For this review, take the finished solid that the model builds, in its own axes (mm). A direction names the side the tool comes from. Give positions to 0.01 mm unless a question says otherwise; leave off trailing zeros. Order: outer loops, then holes, each group sorted by start corner. A loop starts at its lowest first (then second) coordinate and runs counter-clockwise, first axis right, second up.
from build123d import *

# Parameters (mm, degrees)
CYLINDER003_R          = 1.7
CYLINDER003_DEPTH      = 18
CYLINDER003_ROLL_ANGLE = 90.0000000001
CYLINDER002_R          = 3.5
CYLINDER002_DEPTH      = 35
CYLINDER004_R          = 1.5
CYLINDER004_DEPTH      = 40
SKETCH_R               = 4
PAD_DEPTH              = 20
CYLINDER001_R          = 19
CYLINDER001_DEPTH      = 30
CYLINDER001_ROLL_ANGLE = 90.0000000001
CYLINDER_R             = 26.62
CYLINDER_DEPTH         = 40
CYLINDER_ROLL_ANGLE    = 90.0000000001
CUT002_ROLL_ANGLE      = -20


with BuildPart() as cilindro003:
    # Cylinder003 → Cylinder003 (new body)
    with BuildSketch(Plane.XY):
        Circle(CYLINDER003_R)
    extrude(amount=CYLINDER003_DEPTH)


with BuildPart() as cilindro003_1:
    # Cylinder003 roll: moved
    add(cilindro003.part.rotate(Axis((0, 0, 0), (1, 0, 0)), CYLINDER003_ROLL_ANGLE))


with BuildPart() as cilindro003_2:
    # Cylinder003 placement: moved
    add(cilindro003_1.part)


with BuildPart() as cilindro002:
    # Cylinder002 → Cylinder002 (new body)
    with BuildSketch(Plane(origin=(0, -13, 5), x_dir=(1, 0, 0), z_dir=(0, 0, 1))):
        Circle(CYLINDER002_R)
    extrude(amount=CYLINDER002_DEPTH)


with BuildPart() as fusion001:
    # Cylinder004 → Cylinder004 (new body)
    with BuildSketch(Plane(origin=(0, -13, 0), x_dir=(1, 0, 0), z_dir=(0, 0, 1))):
        Circle(CYLINDER004_R)
    extrude(amount=CYLINDER004_DEPTH)

    # Fusion001: union Cilindro003, Cilindro002
    add(cilindro003_2.part)
    add(cilindro002.part)


with BuildPart() as pad:
    # Sketch → Pad (new body, symmetric)
    with BuildSketch(Plane.XZ):
        with Locations((0, 26.6209914966)):
            Circle(SKETCH_R)
        with Locations((14.3923946042, 22.395003144)):
            Circle(SKETCH_R)
        with Locations((24.2153056134, 11.0587595287)):
            Circle(SKETCH_R)
        with Locations((26.3500281875, -3.7885620995)):
            Circle(SKETCH_R)
        with Locations((20.1188029925, -17.4330420298)):
            Circle(SKETCH_R)
        with Locations((7.5, -25.5426542917)):
            Circle(SKETCH_R)
        with Locations((-7.5, -25.5426542917)):
            Circle(SKETCH_R)
        with Locations((-26.3500281875, -3.7885620995)):
            Circle(SKETCH_R)
        with Locations((-24.2153056134, 11.0587595287)):
            Circle(SKETCH_R)
        with Locations((-14.3923946042, 22.395003144)):
            Circle(SKETCH_R)
        with Locations((-20.1188029925, -17.4330420298)):
            Circle(SKETCH_R)
    extrude(amount=PAD_DEPTH, both=True)


with BuildPart() as cilindro001:
    # Cylinder001 → Cylinder001 (new body)
    with BuildSketch(Plane.XY):
        Circle(CYLINDER001_R)
    extrude(amount=CYLINDER001_DEPTH)


with BuildPart() as cilindro001_1:
    # Cylinder001 roll: moved
    add(cilindro001.part.rotate(Axis((0, 0, 0), (1, 0, 0)), CYLINDER001_ROLL_ANGLE))


with BuildPart() as cilindro001_2:
    # Cylinder001 placement: moved
    add(cilindro001_1.part.moved(Location((0, 20, 0))))


with BuildPart() as cut002:
    # Cylinder → Cylinder (new body)
    with BuildSketch(Plane.XY):
        Circle(CYLINDER_R)
    extrude(amount=CYLINDER_DEPTH)


with BuildPart() as cut002_1:
    # Cylinder roll: moved
    add(cut002.part.rotate(Axis((0, 0, 0), (1, 0, 0)), CYLINDER_ROLL_ANGLE))


with BuildPart() as cut002_2:
    # Cylinder placement: moved
    add(cut002_1.part.moved(Location((0, 20, 0))))

    # Cut: cut Cilindro001
    add(cilindro001_2.part, mode=Mode.SUBTRACT)

    # Cut001: cut Pad
    add(pad.part, mode=Mode.SUBTRACT)

    # Cut002: cut Fusion001
    add(fusion001.part, mode=Mode.SUBTRACT)


with BuildPart() as cut002_3:
    # Cut002 roll: moved
    add(cut002_2.part.rotate(Axis((0, 0, 0), (1, 0, 0)), CUT002_ROLL_ANGLE))


with BuildPart() as cut002_4:
    # Cut002 placement: moved
    add(cut002_3.part)


with BuildPart() as part_mirroring008:
    # Part__Mirroring008: instance of Cut002
    add(cut002_4.part.mirror(Plane(origin=(0, 45, 0), x_dir=(1, 0, 0), z_dir=(0, 1, 0))))


solid = part_mirroring008.part
1) Tool access review of faces 1 (the face through (-14.434, 97.387, -21.114)), 2 (the face through (-0.27, 100.76, -0.33)): name each direction out of +Z, -Z, +X, -X, +Y, -Y from which nothing blocks a thin tool from reaching the whole face with its end or side.
Answer sheet:
face 1: -Z, -X, +Y
face 2: none
2) Draft analysis for pull direction Y (two halves, no side actions). For faces 3 (the face through (-7.45, 81, 23.92)), 4 (the face through (-0.373, 108.718, 7.047)), 5 (the face through (10.214, 79.625, 13.273)), state which applies: +Y half, -Y half, draft (parallel to the pull), parting line (faces both ways), or undercut.
Answer sheet:
face 3: -Y half
face 4: +Y half
face 5: undercut
3) We need section A-A on x = 8.5. Give the boundary of the cut face in (y, z), then the cut area to 3 significant figures.
Answer sheet:
outline: (62.58, 16.86) - (65.39, 9.13) - (93.59, 19.39) - (105.21, -12.55) - (77.02, -22.81) - (78.62, -27.2) - (116.21, -13.52) - (100.17, 30.55) - close
area: 856 mm2
4) To check wall thickness, follow line 1 (X direction, y = 85, z = -8.5); line 2 (X direction, y = 101, z = -2); line 3 (Z direction, x = 1, y = 88.5). State the ranges of each line that lie inside material, in increasing order.
Answer sheet:
line 1: x = -23.22 to -17.93, 17.93 to 23.22
line 2: x = -22.81 to -18.14, 18.14 to 22.81
line 3: z = -28.85 to -20.74, 19.65 to 23.66
5) Clearance check with flat-ended pins moving along their axes: pin 1 (3 mm diameter, centred on y = 86, z = -25.5, fed in from -X); pin 2 (3 mm diameter, centred on x = 20, z = -6, fed in from +Y); pin 3 (3 mm diameter, centred on x = 0, z = 12.5, fed in from -Y). State where each tip first meets the part, or that it passes through.
Answer sheet:
pin 1: stops at x = -16.24
pin 2: stops at y = 113.5
pin 3: stops at y = 63.62
